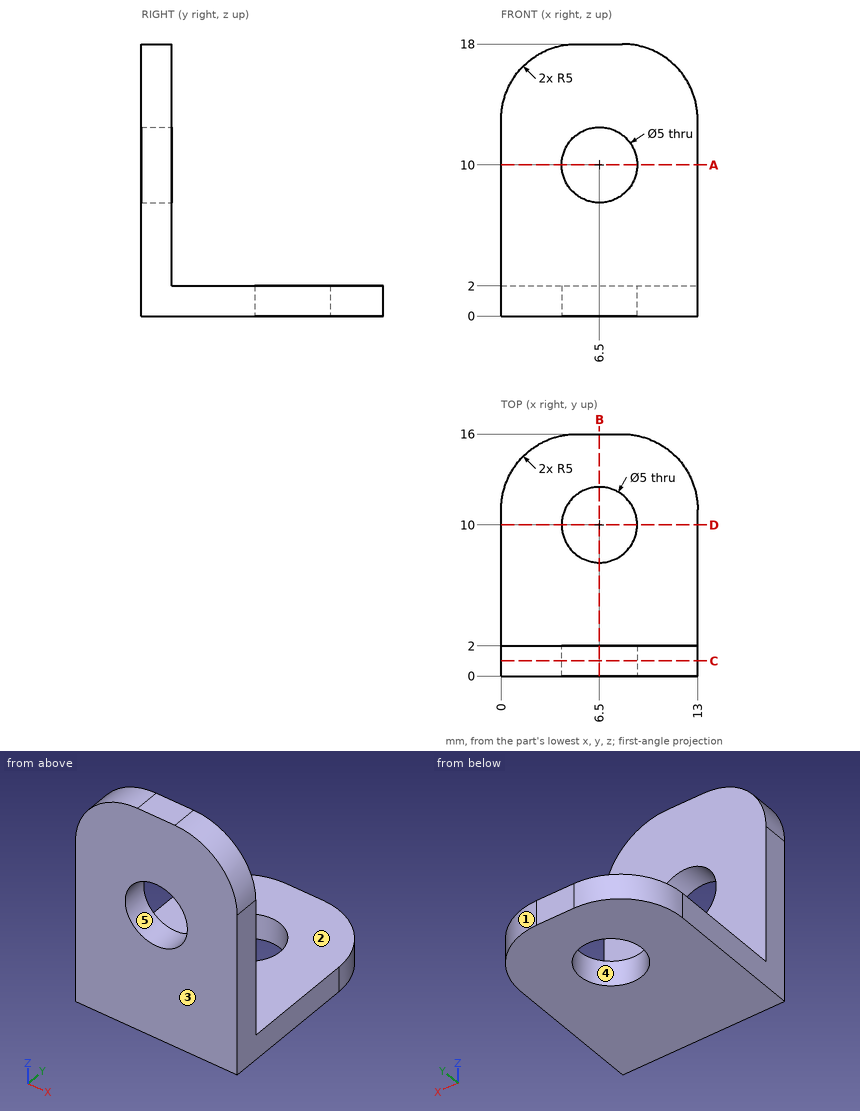
Check sheet for the drawn part. Datum: minimum x, y, z corner. Units: mm. A direction names the side the tool comes from. Give positions to 0.01 mm unless a question says otherwise; leave off trailing zeros. Write each loop counter-clockwise with the first axis right and the second up, starting at its lowest first coordinate (ties: lowest second). Pieces come first, ordered by that corner, then holes. Notation, with made-up numbers: (73.5, 68.25) -> (123.5, 68.25) arc R17 ccw to (123.5, 99.25) -> close; hole circle Ø10 at (24, -2). An arc over 180 degrees is marked (long way). Use one line per item in the form item = value. Start each with the question number.
1. Thickness scan on line 1 along X through (y, z) = (1.2, 10); line 2 along Y through (x, z) = (6.5, 1.25); line 3 along Z through (x, y) = (6.5, 0.7). Record the ranges inside material, lowest first. Write a range as from..to.
2. Section check A-A (z = 10). Record the cut outline in (x, y), and give its area (3 significant figures).
3. Section check C-C (y = 1). Record the cut outline in (x, z), and give its area (3 significant figures).
4. Section check B-B (x = 6.5). Record the cut outline in (y, z).
5. Access from +Z, -Z, +X, -X, +Y, -Y to the whole of each face (thin tool, end or side, straight path). Record for the marked faces 1 and 2.
6. Go/stop test with flat-tipped pins: P1, Ø6.5, axis at x = 6.5, y = 10, coming from the -Z side; P2, Ø4, axis at y = 10, z = 5.5, coming from the +X side; P3, Ø4, axis at x = 4, y = 6.5, coming from the +Z side. Record where each tip stops, or that it passes through.
7. Mould release check, pull along Y, two halves, no side actions. Record for the marked faces 3, 4 and 5: pulls with the +Y half, pulls with the -Y half, needs draft (parallel to the pull), parting line crosses it, or undercut.
Conclusion:
q1.line_1 = 0..4, 9..13
q1.line_2 = 0..7.5, 12.5..16
q1.line_3 = 0..7.5, 12.5..18
q2.outline = (0, 0) -> (4, 0) -> (4, 2) -> (0, 2) -> close; (9, 0) -> (13, 0) -> (13, 2) -> (9, 2) -> close
q2.area = 16.0 mm²
q3.outline = (0, 0) -> (13, 0) -> (13, 13) arc R5 ccw to (8, 18) -> (5, 18) arc R5 ccw to (0, 13) -> close; hole circle Ø5 at (6.5, 10)
q3.area = 204 mm²
q4.outline = (0, 0) -> (7.5, 0) -> (7.5, 2) -> (2, 2) -> (2, 7.5) -> (0, 7.5) -> close; (0, 12.5) -> (2, 12.5) -> (2, 18) -> (0, 18) -> close; (12.5, 0) -> (16, 0) -> (16, 2) -> (12.5, 2) -> close
q5.face_1 = +Z, -Z, +X, +Y
q5.face_2 = +Z, +X, -X, +Y
q6.P1 = 0
q6.P2 = through
q6.P3 = 2
q7.face_3 = pulls with the -Y half
q7.face_4 = undercut
q7.face_5 = needs draft
